Input: dimensioned drawing with shaded views. Units: mm. Origin: part minimum x, y, z. A direction names the side the tool comes from. Coordinates: 2 decimals unless noted, no trailing zeros. Loops run counter-clockwise (first coordinate to the right, second up) from the corner with the lowest first, then second, coordinate; pieces in that order, holes last. Notation, with made-up numbers: (31, 32) - (73, 32) arc R21 cw to (73, 41) - close; hole circle Ø8 at (11, -34). An arc over 180 degrees is marked (long way). Put each result on its own line as item: value. Start each with the question number.
1) Material intervals for line 1 along Y through (x, z) = (2.1, 7.62); line 2 along Z through (x, y) = (18.25, 14) (1 decimal); line 3 along X through (y, z) = (14.75, 31) (1 decimal), sorted ascending. Write a range as from..to.
2) Reachability of the marked faces 1, 2 and 3 from +Z, -Z, +X, -X, +Y, -Y: full face, straight path, thin tool, end or side. Return the list, or none.
3) Section A-A on z = 7.62. Count the separate pieces of the cut face and the enclosed holes in it.
4) Section C-C on y = 16.75. Output: boundary loops of the cut face in (x, z) (1 decimal).
5) Contact query for flat-ended pins moving along their axis: pin 1 Ø5.5 at (x, y) = (8, 5.5) entering from -Z; pin 2 Ø2 at (x, y) = (12.065, 9.525) entering from -Z; pin 3 Ø3 at (y, z) = (4.13, 7.62) entering from +X (1 decimal); pin 4 Ø1 at (x, y) = (5.5, 2) entering from +Z. Output: stop coordinate, or through.
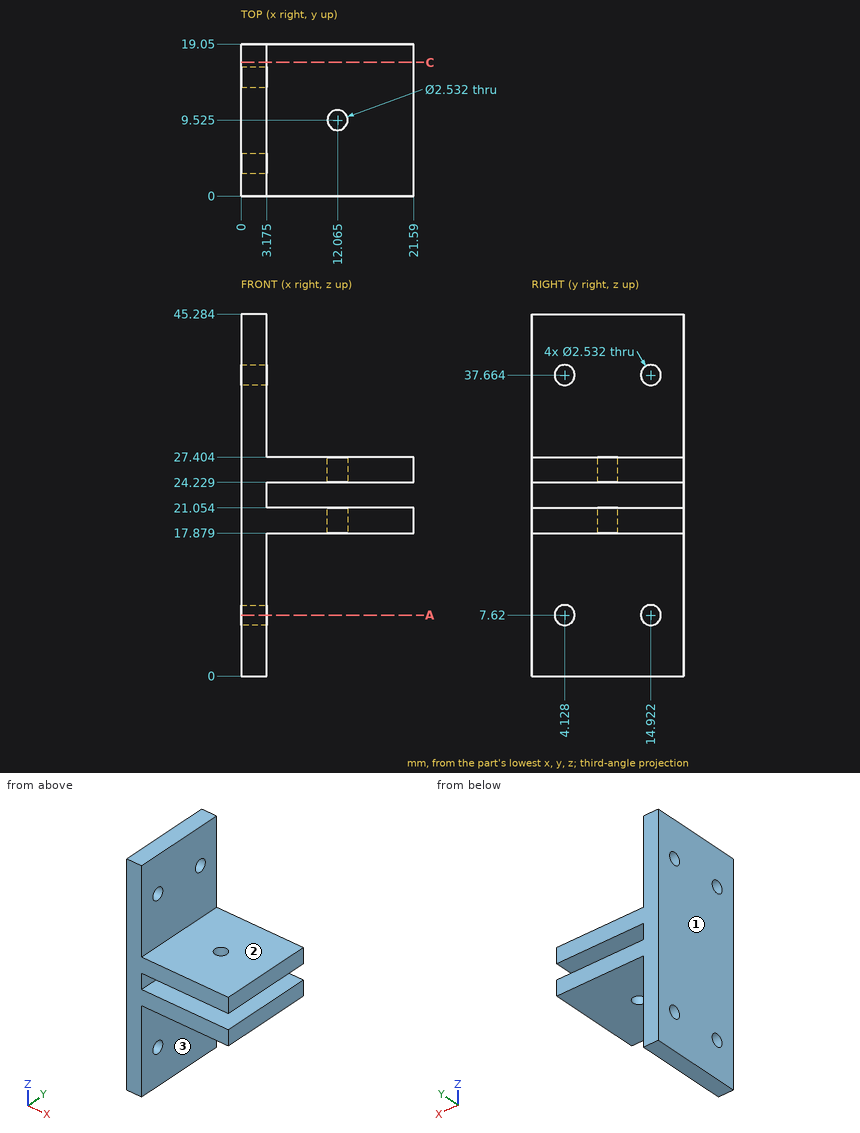
Answer block:
1. line 1: y = 0..2.86, 5.39..13.66, 16.19..19.05
1. line 2: z = 17.9..21.1, 24.2..27.4
1. line 3: x = 0..3.2
2. face 1: +Z, -Z, -X, +Y, -Y
2. face 2: +Z, +X, +Y, -Y
2. face 3: -Z, +X, +Y, -Y
3. separate pieces: 3
3. enclosed holes: 0
4. outline: (0, 0) - (3.2, 0) - (3.2, 17.9) - (21.6, 17.9) - (21.6, 21.1) - (3.2, 21.1) - (3.2, 24.2) - (21.6, 24.2) - (21.6, 27.4) - (3.2, 27.4) - (3.2, 45.3) - (0, 45.3) - close
5. pin 1: stops at z = 17.88
5. pin 2: passes through
5. pin 3: stops at x = 3.2
5. pin 4: stops at z = 27.4
